Verification items for the finished model (mm, model axes). Face numbers are marked on the shaded views. A direction names the side the tool comes from. Round coordinates to 2 decimals unless told otherwise and drop trailing zeros. Write each loop counter-clockwise with the first axis right and the second up, starting at its lowest first coordinate (ties: lowest second). Pieces come first, ordered by that corner, then holes. Notation, with made-up numbers: M -19,70 L -15,70 A20 cw -15,79 Z; hole C 38.25,-22 d1. An arc over 180 degrees is marked long. One line per item, written item: value. Start each with the question number.
Autodesk Inventor part; units mm, degrees
ref_plane "YZ Plane" through (0, 0, 0) normal (1, 0, 0) x (0, 1, 0)
ref_plane "XZ Plane" through (0, 0, 0) normal (0, 1, 0) x (-1, 0, 0)
ref_plane "XY Plane" through (0, 0, 0) normal (0, 0, 1) x (1, 0, 0)
sketch "Sketch2" plane through (0, 0, 0) normal (0, 0, 1) x (1, 0, 0)
  arc A0 (-35.8105, 1.2215) -> (-35.8105, -1.2215) centre (-34.7965, 0) ccw
  arc A1 (35.4376, -1.3856) -> (35.4495, 1.0387) centre (34.4185, -0.1685) ccw
  line L0 (-35.8105, 1.2215) -> (-15.2094, 18.3224)
  line L1 (-35.8105, -1.2215) -> (-15.2094, -18.3224)
  line L2 (-73.8497, 0) -> (129.1726, 0) construction
  line L3 (15.465, 18.1071) -> (35.4495, 1.0387)
  line L4 (35.4376, -1.3856) -> (15.2871, -18.2576)
  line L5 (-36.384, 17.9881) -> (-36.384, -16.5847) construction
  line L6 (36.006, 40.1283) -> (36.006, -35.2466) construction
  circle A2 centre (-23.8125, 0) radius 2.4892
  circle A3 centre (23.8125, 0) radius 2.4892
  circle A4 centre (0, 0) radius 11.8999
  arc A5 (-15.2094, -18.3224) -> (15.2871, -18.2576) centre (0, 0) ccw
  arc A6 (15.465, 18.1071) -> (-15.2094, 18.3224) centre (0, 0) ccw
  dimension "d6" = 3.175
  dimension "d7" = 72.39
  dimension "d8" = 23.7998
  dimension "d9" = 4.9784
extrude "Extrusion1" add sketch "Sketch2" along normal blind 3.175
sketch "Sketch3" plane through (0, 0, 0) normal (0, 0, -1) x (-1, 0, 0)
  circle A0 centre (0, 0) radius 19.05
  circle A1 centre (0, 0) radius 11.8999
  dimension "d12" = 38.1
extrude "Extrusion2" add sketch "Sketch3" along normal blind 25.146
sketch "Sketch4" plane through (0, 0, -25.146) normal (0, 0, -1) x (-1, 0, 0)
  circle A0 centre (0, 0) radius 11.8999
  circle A1 centre (0, 0) radius 14.2621
  dimension "d15" = 28.5242
extrude "Extrusion3" add sketch "Sketch4" along normal blind 6.35
sketch "Sketch5" plane through (0, 0, 3.175) normal (0, 0, 1) x (1, 0, 0)
  circle A0 centre (0, 0) radius 11.8999
  circle A1 centre (0, 0) radius 15.875
  dimension "d18" = 31.75
extrude "Extrusion4" cut sketch "Sketch5" against normal blind 1.6002
sketch "Sketch6" plane through (0, 0, 1.5748) normal (0, 0, 1) x (1, 0, 0)
  circle A0 centre (0, 0) radius 14.2748
  circle A1 centre (0, 0) radius 11.8999
  dimension "d21" = 28.5496
extrude "Extrusion5" cut sketch "Sketch6" against normal blind 9.525
properties part number "Bearing Block WCP"
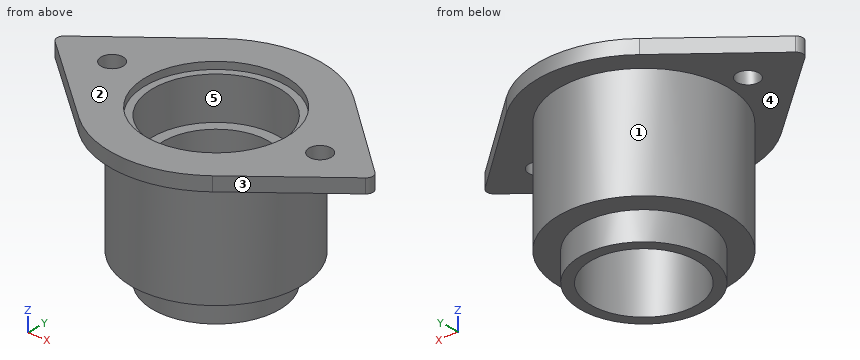
1) Cross-section at B-B (y = -4). Record the boundary of the cut face in (x, z) (3 decimals), then the cut area to 3 significant figures.
2) Cross-section at A-A (x = 0). Record the boundary of the cut face in (y, z) (3 decimals), then the cut area to 3 significant figures.
3) Cross-section at D-D (y = -13). Record the boundary of the cut face in (x, z) (3 decimals).
4) Thickness scan on line 1 (Y direction, x = 0, z = 2) (3 decimals); line 2 (Y direction, x = 0, z = -20); line 3 (Z direction, x = 29.5, y = -1) (3 decimals). Record the ranges inside material, lowest first.
5) Access from +Z, -Z, +X, -X, +Y, -Y to the whole of each face (thin tool, end or side, straight path). Record for the marked faces 1 and 2.
6) Gauge pin test, flat ends, axial feed: pin 1 Ø4 at (x, z) = (15, -19) entering from -Y; pin 2 Ø5 at (x, y) = (14, -15.5) entering from -Z; pin 3 Ø17 at (x, y) = (0, 0) entering from -Z; pin 4 Ø5.5 at (x, y) = (23.81, 0) entering from -Z. Record the tip position at first contact, or that the pin passes through.
7) Cross-section at C-C (z = -3). Record the boundary of the cut face in (x, y).
8) Mould release check, pull along Y, two halves, no side actions. Record for the marked faces 3, 4 and 5: pulls with the +Y half, pulls with the -Y half, needs draft (parallel to the pull), parting line crosses it, or undercut.
Results below:
1. outline: M -32.463,0 L -18.625,0 L -18.625,-25.146 L -13.69,-25.146 L -13.69,-31.496 L -11.207,-31.496 L -11.207,-7.95 L -13.703,-7.95 L -13.703,1.575 L -15.363,1.575 L -15.363,3.175 L -32.463,3.175 Z; M 11.207,-31.496 L 13.69,-31.496 L 13.69,-25.146 L 18.625,-25.146 L 18.625,0 L 32.315,0 L 32.315,3.175 L 15.363,3.175 L 15.363,1.575 L 13.703,1.575 L 13.703,-7.95 L 11.207,-7.95 Z
1. area: 478 mm²
2. outline: M -23.813,0 L -19.05,0 L -19.05,-25.146 L -14.262,-25.146 L -14.262,-31.496 L -11.9,-31.496 L -11.9,-7.95 L -14.275,-7.95 L -14.275,1.575 L -15.875,1.575 L -15.875,3.175 L -23.813,3.175 Z; M 11.9,-31.496 L 14.262,-31.496 L 14.262,-25.146 L 19.05,-25.146 L 19.05,0 L 23.812,0 L 23.812,3.175 L 15.875,3.175 L 15.875,1.575 L 14.275,1.575 L 14.275,-7.95 L 11.9,-7.95 Z
2. area: 407 mm²
3. outline: M -21.621,0 L -13.925,0 L -13.925,-25.146 L -5.866,-25.146 L -5.866,-31.496 L 5.866,-31.496 L 5.866,-25.146 L 13.925,-25.146 L 13.925,0 L 21.566,0 L 21.566,3.175 L 9.111,3.175 L 9.111,1.575 L 5.897,1.575 L 5.897,-7.95 L -5.897,-7.95 L -5.897,1.575 L -9.111,1.575 L -9.111,3.175 L -21.621,3.175 Z
4. line 1: y = -23.813 to -15.875, 15.875 to 23.812
4. line 2: y = -19.05 to -11.9, 11.9 to 19.05
4. line 3: z = 0 to 3.175
5. face 1: -Z
5. face 2: +Z, +X, -X, +Y, -Y
6. pin 1: stops at y = -13.92
6. pin 2: stops at z = -25.15
6. pin 3: passes through
6. pin 4: stops at z = 0
7. outline: C 0,0 d38.1; hole C 0,0 d28.55
8. face 3: pulls with the -Y half
8. face 4: needs draft
8. face 5: undercut
